Could you check a few things on this drawing? It's one solid part, dimensions in mm from its lowest x, y, z. A direction names the side the tool comes from. Give positions to 0.01 mm unless a question says otherwise; leave off trailing zeros. Write each loop counter-clockwise with the first axis right and the second up, starting at its lowest first coordinate (ties: lowest second). Pieces come first, ordered by that corner, then holes. Notation, with made-up numbers: (-27, -17.5) -> (28, -17.5) arc R10 ccw to (28, -12.5) -> close; hole circle Ø3 at (-15, 8). An arc over 180 degrees is marked (long way). Use CSV: the item, a comma, the result in double quotes. Start each with the question number.
(1) Which directions (+Z, -Z, +X, -X, +Y, -Y) give clear straight access to the entire face, cutting with the end or side of a thin tool? Please do the marked faces 1 and 2.
(2) Suppose I cut it at C-C on x = 9. List the corners of the cut face in (y, z) for me, plus the area to 3 significant figures.
(3) I need wall thicknesses on L1, parallel to Y at x = 12.7, z = 3.25; L2, parallel to Y at x = 13.25, z = 2.75; L3, parallel to X at y = 12, z = 5.5. Which ranges of each line are inside material? Lowest first, please. Write a range as [from, to].
(4) For pin 1 Ø2.5 at (x, z) = (3, 3.25) entering from +Y; pin 2 Ø3.5 at (y, z) = (16.65, 3.25) entering from -X; pin 3 Ø1 at (x, z) = (5, 5.5) entering from +Y, each with a flat end and sliding along its axis, tell me the tip position at first contact or that it passes through.
(5) Suppose I cut it at D-D on x = 13.5. List the corners of the cut face in (y, z) for me, plus the area to 3 significant figures.
(6) Suppose I cut it at B-B on z = 3.25. List the corners of the cut face in (x, y) for me.
(7) If we mould it in two halves opening along Y, with no side actions, what happens to the marked faces 3, 4 and 5? For each: pulls with the +Y half, pulls with the -Y half, needs draft (parallel to the pull), parting line crosses it, or undercut.
(8) Suppose I cut it at A-A on y = 7.35. List the corners of the cut face in (x, z) for me, plus the area to 3 significant figures.
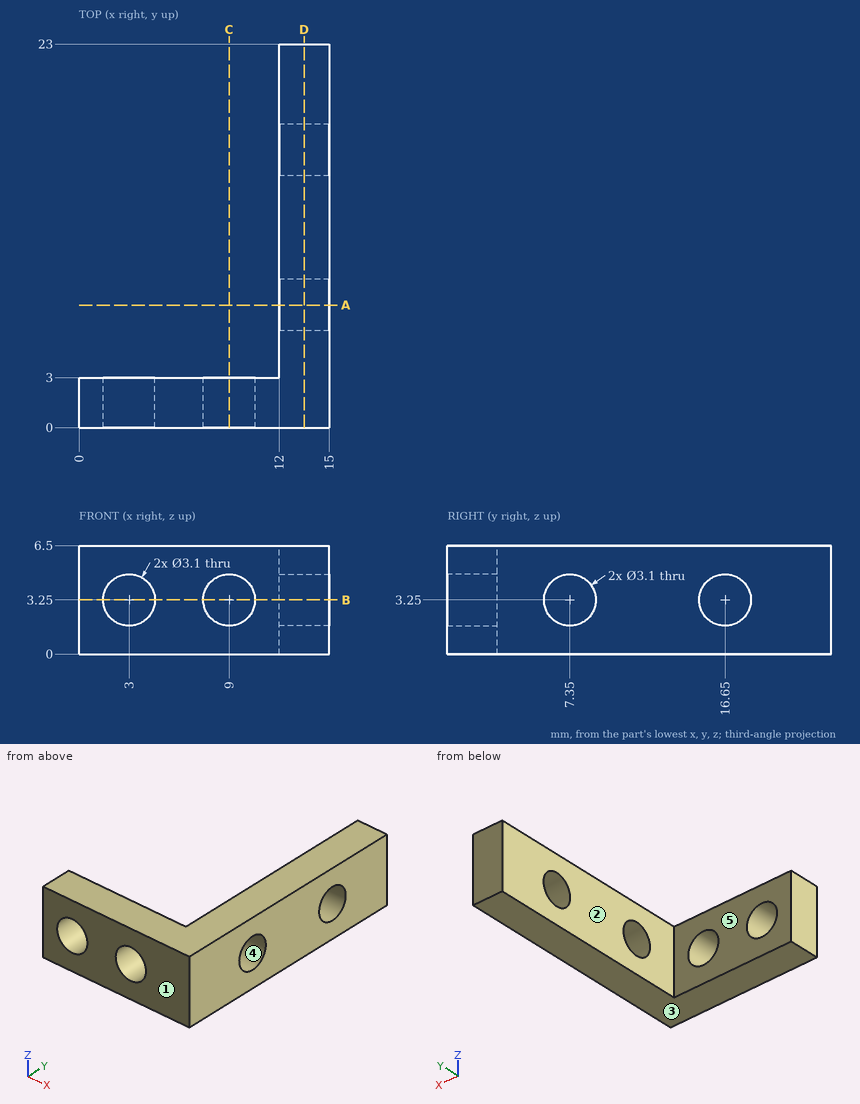
Geometry says:
1,face 1,"+Z, -Z, +X, -X, -Y"
1,face 2,"+Z, -Z, -X, +Y"
2,outline,"(0, 0) -> (3, 0) -> (3, 1.7) -> (0, 1.7) -> close; (0, 4.8) -> (3, 4.8) -> (3, 6.5) -> (0, 6.5) -> close"
2,area,"10.2 mm²"
3,L1,"[0, 5.8], [8.9, 15.1], [18.2, 23]"
3,L2,"[0, 5.88], [8.82, 15.18], [18.12, 23]"
3,L3,"[12, 15]"
4,pin 1,"through"
4,pin 2,"x = 12"
4,pin 3,"y = 3"
5,outline,"(0, 0) -> (23, 0) -> (23, 6.5) -> (0, 6.5) -> close; hole circle Ø3.1 at (7.35, 3.25); hole circle Ø3.1 at (16.65, 3.25)"
5,area,"134 mm²"
6,outline,"(0, 0) -> (1.45, 0) -> (1.45, 3) -> (0, 3) -> close; (4.55, 0) -> (7.45, 0) -> (7.45, 3) -> (4.55, 3) -> close; (10.55, 0) -> (15, 0) -> (15, 5.8) -> (12, 5.8) -> (12, 3) -> (10.55, 3) -> close; (12, 8.9) -> (15, 8.9) -> (15, 15.1) -> (12, 15.1) -> close; (12, 18.2) -> (15, 18.2) -> (15, 23) -> (12, 23) -> close"
7,face 3,"needs draft"
7,face 4,"undercut"
7,face 5,"pulls with the +Y half"
8,outline,"(12, 0) -> (15, 0) -> (15, 1.7) -> (12, 1.7) -> close; (12, 4.8) -> (15, 4.8) -> (15, 6.5) -> (12, 6.5) -> close"
8,area,"10.2 mm²"
